Drawing for the job (mm, zero at the part's lowest x, y, z). A direction names the side the tool comes from. Coordinates: 2 decimals unless noted, no trailing zeros. Write each loop counter-clockwise with the first axis right and the second up, starting at its lowest first coordinate (ties: lowest second). Pieces come first, ordered by that corner, then holes. Notation, with made-up numbers: M 38.25,50 L 90.25,50 A24 ccw 90.25,77 Z; hole C 30.25,35 d4. An arc over 180 degrees is marked long. Use a Markdown table: item, result. Add a question column.
Q1. Tool access for the marked faces 1 and 2: list every direction of +Z, -Z, +X, -X, +Y, -Y with a clear straight run to the whole face (end or side of a thin tool).
Q2. Slice it at B-B on x = 31.75. Write the cut outline in (y, z).
Q3. Slice it at A-A on y = 19.05. Write the cut outline in (x, z).
Q4. Slice it at D-D on z = 18.5. Write the cut outline in (x, y), then the cut area to 3 significant figures.
Q5. Wall check: L1, parallel to Y at x = 31.75, z = 33; L2, parallel to X at y = 19.05, z = 33.5; L3, parallel to Z at x = 14, y = 72. Give the ranges that are in metal, low to high. Write a range as from..to.
Q6. Pin check, flat tips, straight feed: pin 1 Ø3 at (x, z) = (8, 11) entering from +Y; pin 2 Ø1.5 at (y, z) = (116, 27.5) entering from -X; pin 3 Ø1 at (x, y) = (34, 28.5) entering from -Z; pin 4 Ø10.5 at (y, z) = (25.4, 11.1) entering from +X. Stop position of each tip, or through.
Q7. Slice it at C-C on y = 107. Write the cut outline in (x, z), then the cut area to 3 significant figures.
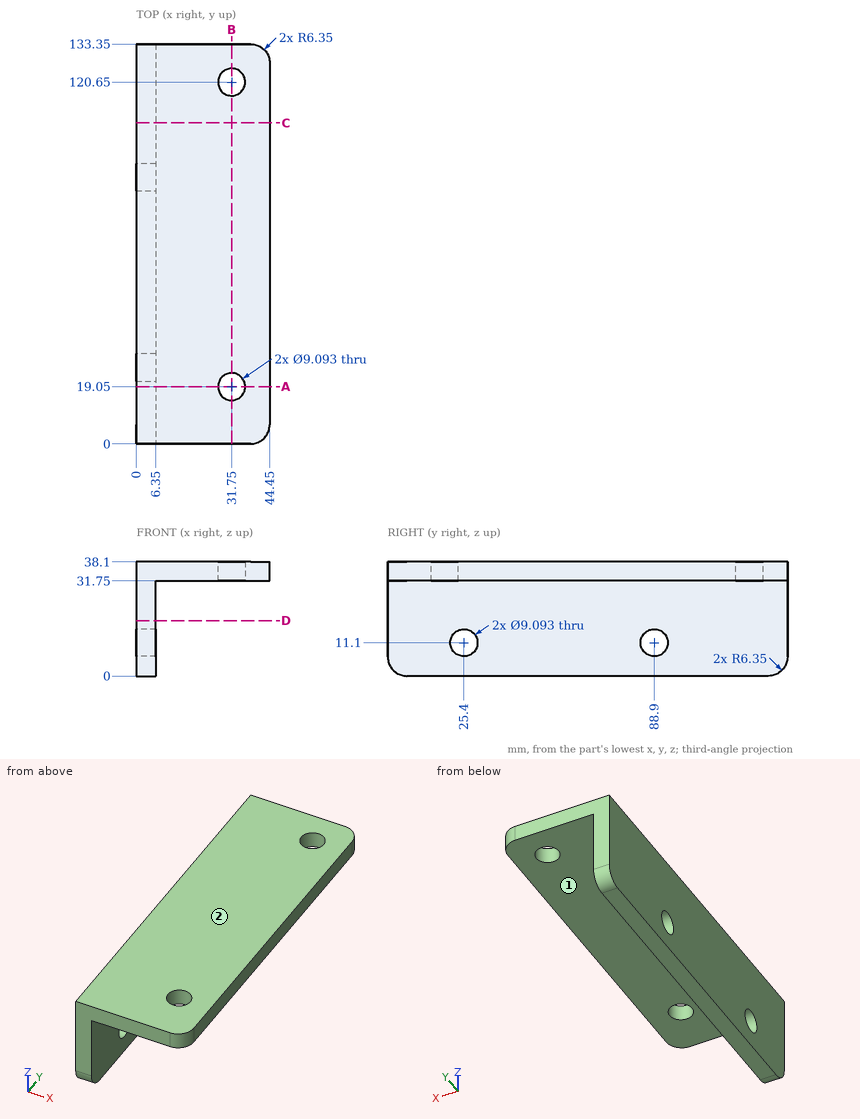
Recorded:
| question | item | result |
|---|---|---|
| 1 | face 1 | -Z, +X, +Y, -Y |
| 1 | face 2 | +Z, +X, -X, +Y, -Y |
| 2 | outline | M 0,31.75 L 14.5,31.75 L 14.5,38.1 L 0,38.1 Z; M 23.6,31.75 L 116.1,31.75 L 116.1,38.1 L 23.6,38.1 Z; M 125.2,31.75 L 133.35,31.75 L 133.35,38.1 L 125.2,38.1 Z |
| 3 | outline | M 0,0 L 6.35,0 L 6.35,31.75 L 27.2,31.75 L 27.2,38.1 L 0,38.1 Z; M 36.3,31.75 L 44.45,31.75 L 44.45,38.1 L 36.3,38.1 Z |
| 4 | outline | M 0,0 L 6.35,0 L 6.35,133.35 L 0,133.35 Z |
| 4 | area | 847 mm² |
| 5 | L1 | 0..14.5, 23.6..116.1, 125.2..133.35 |
| 5 | L2 | 0..27.2, 36.3..44.45 |
| 5 | L3 | 31.75..38.1 |
| 6 | pin 1 | through |
| 6 | pin 2 | x = 0 |
| 6 | pin 3 | z = 31.75 |
| 6 | pin 4 | x = 6.35 |
| 7 | outline | M 0,0 L 6.35,0 L 6.35,31.75 L 44.45,31.75 L 44.45,38.1 L 0,38.1 Z |
| 7 | area | 484 mm² |
